from build123d import *

# Parameters (mm, degrees)
SKETCH1_W           = 33
SKETCH1_H           = 10
BOSS_EXTRUDE1_DEPTH = 1
SKETCH3_W           = 5
SKETCH3_H           = 5
BOSS_EXTRUDE2_DEPTH = 1.2
LPATTERN1_COUNT     = 8
LPATTERN1_PITCH     = 33
LPATTERN1_COL_COUNT = 7
LPATTERN1_COL_PITCH = 33


with BuildPart() as part:
    # Sketch1 → Boss-Extrude1 (new body)
    with BuildSketch(Plane(origin=(0, 0, 0), x_dir=(1, 0, 0), z_dir=(0, 1, 0))):
        Rectangle(SKETCH1_W, SKETCH1_H)
    boss_extrude1 = extrude(amount=BOSS_EXTRUDE1_DEPTH)

    # Sketch3 → Boss-Extrude2 (add)
    with BuildSketch(Plane(origin=(0, 1, 0), x_dir=(1, 0, 0), z_dir=(0, 1, 0))):
        Rectangle(SKETCH3_W, SKETCH3_H)
    boss_extrude2 = extrude(amount=BOSS_EXTRUDE2_DEPTH)

    # LPattern1: Boss-Extrude1, Boss-Extrude2 ×8
    with Locations(*[(-i * LPATTERN1_PITCH, 0, 0) for i in range(1, LPATTERN1_COUNT)]):
        add(boss_extrude1)
        add(boss_extrude2)

    # LPattern1 col: Boss-Extrude1, Boss-Extrude2 ×7
    with Locations(*[(i * LPATTERN1_COL_PITCH, 0, 0) for i in range(1, LPATTERN1_COL_COUNT)]):
        add(boss_extrude1)
        add(boss_extrude2)


solid = part.part
Build history of the part. All positions in model axes, mm. Coordinates: 2 decimals unless noted, no trailing zeros. Write each loop counter-clockwise with the first axis right and the second up, starting at its lowest first coordinate (ties: lowest second). Pieces come first, ordered by that corner, then holes. Notation, with made-up numbers: (45, 55.5) -> (73, 55.5) arc R14 ccw to (73, 79.5) -> close; hole circle Ø8 at (-6, -29). An arc over 180 degrees is marked (long way). Use CSV: the item, a comma, the result in double quotes. Start each with the question number.
Q1. Cut at A-A, the plane y = 1.75. State how many separate pieces and enclosed holes the cut face has, then the cut area to 3 significant figures.
Q2. Cut at B-B, the plane x = 117.5. List the corners of the cut face in (y, z).
Q3. Drill centre lines: probe 1 along Z at (x, y) = (-1.5, 1.7); probe 2 along Y at (x, z) = (-2.5, -4.5). Where is each one in solid material? Low to high.
Q4. Pull direction X, two halves, no side cores. Call faces 1 (the flat face through (-20, 1, 0)), 2 (the flat face through (-20, 0, 0)): released by +X, released by -X, zero draft, split by the parting line, or undercut.
Q5. Flat gauge pins, fed straight in: pin 1 Ø1.3 at (y, z) = (2, -1) entering from +X; pin 2 Ø0.6 at (y, z) = (1.5, -1) entering from -X; pin 3 Ø5 at (x, z) = (-7.5, 1.5) entering from +Y. Where does each tip first touch, or does it go through?
Checked values:
1,separate pieces,"14"
1,enclosed holes,"0"
1,area,"350 mm²"
2,outline,"(0, -5) -> (1, -5) -> (1, 5) -> (0, 5) -> close"
3,probe 1,"z = -2.5 to 2.5"
3,probe 2,"y = 0 to 1"
4,face 1,"undercut"
4,face 2,"zero draft"
5,pin 1,"stops at x = 200.5"
5,pin 2,"stops at x = -233.5"
5,pin 3,"stops at y = 1"
